Source: three-view drawing plus pictorial views. Frame: mm from the lowest corner of the part. A direction names the side the tool comes from. Round coordinates to 2 decimals unless told otherwise and drop trailing zeros. Loops run counter-clockwise (first coordinate to the right, second up) from the corner with the lowest first, then second, coordinate; pieces in that order, holes last. Notation, with made-up numbers: M 86,-35.75 L 145,-35.75 A30 ccw 145,-11.75 Z; hole C -22.5,83.5 d11. An arc over 180 degrees is marked long. Answer as a JSON object with one key per item and string values.
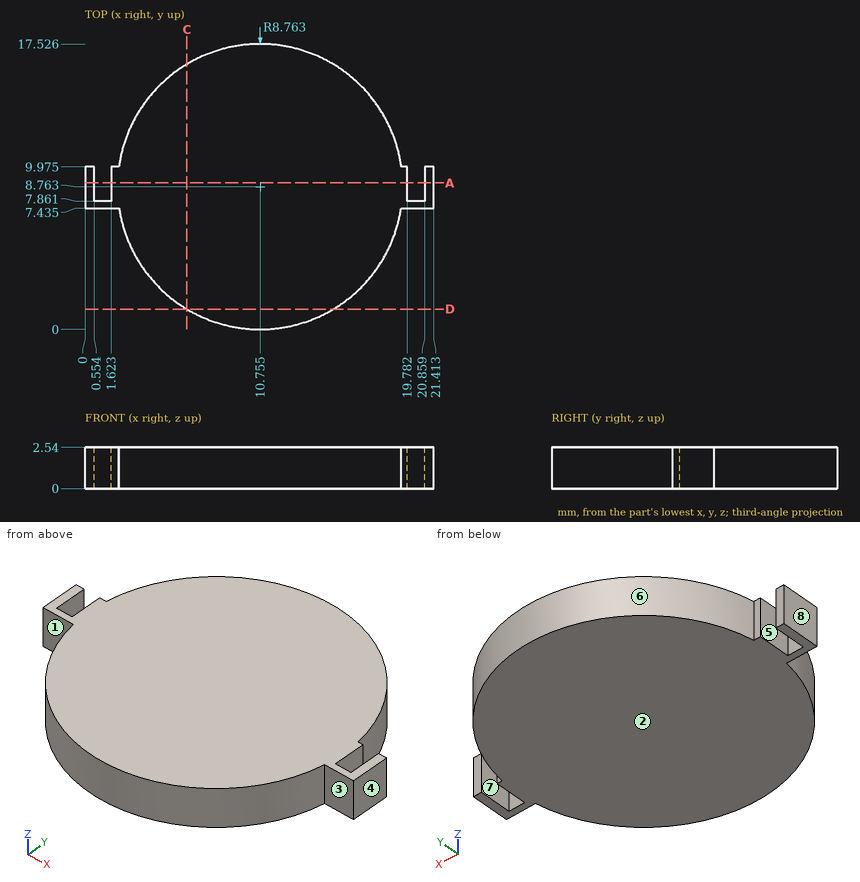
1) Line query: probe 1 along X at (y, z) = (8, 1.95); probe 2 along Y at (x, z) = (10.5, 0.75); probe 3 along Y at (x, z) = (19.5, 2) (1 decimal). Output: solid intervals per line, ascending.
Geometry results:
{"probe 1": "0 to 0.55, 1.62 to 19.78, 20.86 to 21.41", "probe 2": "0 to 17.52", "probe 3": "7.4 to 10"}
2) Cut plane C-C on x = 6.25. Return the cut outline in (y, z).
Geometry results:
{"outline": "M 1.25,0 L 16.28,0 L 16.28,2.54 L 1.25,2.54 Z"}
3) Set-up query: the marked faces 1, 2, 3, 4 and 5. Return all of +Z, -Z, +X, -X, +Y, -Y with unobstructed straight access to the full face (end or side cutting, diameter ignored); none if empty.
Geometry results:
{"face 1": "+Z, -Z, -X, -Y", "face 2": "-Z, +X, -X, +Y, -Y", "face 3": "+Z, -Z, +X, -Y", "face 4": "+Z, -Z, +X, +Y, -Y", "face 5": "+Z, -Z, +Y"}
4) Pull-direction query (X, two-part tool) for the marked faces 6, 7 and 8; classes: +X half, -X half, draft (parallel to the pull), parting line (faces both ways), or undercut.
Geometry results:
{"face 6": "parting line", "face 7": "undercut", "face 8": "-X half"}
5) Cut plane D-D on y = 1.25. Return the cut outline in (x, z) (1 decimal).
Geometry results:
{"outline": "M 6.2,0 L 15.3,0 L 15.3,2.5 L 6.2,2.5 Z"}
6) Cut plane A-A on y = 9. Return the cut outline in (x, z).
Geometry results:
{"outline": "M 0,0 L 0.55,0 L 0.55,2.54 L 0,2.54 Z; M 1.62,0 L 19.78,0 L 19.78,2.54 L 1.62,2.54 Z; M 20.86,0 L 21.41,0 L 21.41,2.54 L 20.86,2.54 Z"}
7) First-contact query: pin 1 (0.6 mm diameter, centred on x = 1, z = 1.5, fed in from -Y) (1 decimal); pin 2 (0.5 mm diameter, centred on x = 1, z = 0.5, fed in from +Y); pin 3 (0.9 mm diameter, centred on x = 20.5, z = 1.5, fed in from +Y) (1 decimal). Flat tips, straight axial feed; report the tip coordinate or a pass-through.
Geometry results:
{"pin 1": "y = 7.4", "pin 2": "y = 7.86", "pin 3": "y = 10"}
